Verification items for the finished model (mm, model axes). A direction names the side the tool comes from. Round coordinates to 2 decimals unless told otherwise and drop trailing zeros. Order: outer loops, then holes, each group sorted by start corner. A loop starts at its lowest first (then second) coordinate and runs counter-clockwise, first axis right, second up.
```python
from build123d import *

# Parameters (mm, degrees)
SKETCH1_W           = 104
SKETCH1_H           = 9.72
BODY_DEPTH          = 17.75
FRONT_CUT_OUT_DEPTH = 89.865925518
SKETCH4_R           = 3.5
BOSS_EXTRUDE2_DEPTH = 9.5


with BuildPart() as part:
    # Sketch1 → body (new body)
    with BuildSketch(Plane.XY):
        with Locations((34.530987618, 4.261078665)):
            Rectangle(SKETCH1_W, SKETCH1_H)
    extrude(amount=BODY_DEPTH)

    # Sketch2 → front_cut_out (cut, through all)
    with BuildSketch(Plane.XZ.offset(0.598921335)):
        with BuildLine():
            Line((46.030987618, 17.75), (56.030987618, 14.8))
            Line((56.030987618, 14.8), (80.030987618, 14.8))
            ThreePointArc((80.030987618, 14.8), (85.955987618, 8.875), (80.030987618, 2.95))
            Line((80.030987618, 2.95), (56.030987618, 2.95))
            Line((56.030987618, 2.95), (46.030987618, 0))
            Line((46.030987618, 0), (86.530987618, 0))
            Line((86.530987618, 0), (86.530987618, 17.75))
            Line((86.530987618, 17.75), (46.030987618, 17.75))
        make_face()
    extrude(amount=-FRONT_CUT_OUT_DEPTH, mode=Mode.SUBTRACT)

    # Sketch4 → Boss-Extrude2 (add)
    with BuildSketch(Plane.XZ.offset(0.598921335)):
        with Locations(Location((-8.469012382, 8.875, 0), (0, 0, 180))):
            Circle(SKETCH4_R)
        with Locations(Location((42.530987618, 8.875, 0), (0, 0, 180))):
            Circle(SKETCH4_R)
        with Locations(Location((59.530872729, 9, 0), (0, 0, 180))):
            Circle(SKETCH4_R)
        with Locations(Location((76.530895707, 9, 0), (0, 0, 180))):
            Circle(SKETCH4_R)
    extrude(amount=BOSS_EXTRUDE2_DEPTH)


solid = part.part
```
1) Sectioned sample at D-D on z = 16. Record the cut outline in (x, y), then the cut area to 3 significant figures.
2) Draft check along X on faces 1 (the flat face through (51.101, 4.193, 1.496)), 2 (the cylindrical face through (73.298, -5.282, 10.341)), 3 (the flat face through (43, -10.099, 9)), 4 (the flat face through (-17.469, 4, 9)). Enter one of: released by +X, released by -X, zero draft, split by the parting line, or undercut.
3) Scan lines: probe 1 along X at (y, z) = (-8, 6.75); probe 2 along Y at (x, z) = (53, 12); probe 3 along Z at (x, y) = (42.5, -8.5). Record each from-to range of solid material in increasing order.
4) Sectioned sample at B-B on x = 60.5. Record the cut outline in (y, z), then the cut area to 3 significant figures.
5) Sectioned sample at A-A on y = 6.5. Record the cut outline in (x, z) (3 decimals).
6) Tool access check on faces 5 (the flat face through (68, 4, 14.8)), 6 (the cylindrical face through (39.3, -5.28, 10.22)), 7 (the flat face through (77, -10.099, 9)), 8 (the flat face through (68, 4, 2.95)), 9 (the cylindrical face through (85.955, 4.193, 9.005)). Record the directions out of +Z, -Z, +X, -X, +Y, -Y that give a thin tool (end or side, any length) a straight path to the whole face; none if there is none.
7) Sectioned sample at C-C on y = -1.5. Record the cut outline in (x, z) (3 decimals).
8) Go/stop test with flat-tipped pins: pin 1 Ø5 at (x, y) = (64.5, -0.5) entering from +Z; pin 2 Ø5 at (x, y) = (60, 2) entering from -Z; pin 3 Ø1.5 at (y, z) = (-0.5, 13) entering from +X. Record where each tip stops, or that it passes through.
Returned:
1. outline: (-17.47, -0.6) - (51.96, -0.6) - (51.96, 9.12) - (-17.47, 9.12) - close
1. area: 675 mm2
2. face 1: released by +X
2. face 2: undercut
2. face 3: zero draft
2. face 4: released by -X
3. probe 1: x = -11.25 to -5.69, 39.75 to 45.31, 56.85 to 62.21, 73.85 to 79.21
3. probe 2: y = -0.6 to 9.12
3. probe 3: z = 5.38 to 12.37
4. outline: (-10.1, 5.64) - (-0.6, 5.64) - (-0.6, 2.95) - (9.12, 2.95) - (9.12, 14.8) - (-0.6, 14.8) - (-0.6, 12.36) - (-10.1, 12.36) - close
4. area: 179 mm2
5. outline: (-17.469, 0) - (46.031, 0) - (56.031, 2.95) - (80.031, 2.95) arc R5.925 ccw to (80.031, 14.8) - (56.031, 14.8) - (46.031, 17.75) - (-17.469, 17.75) - close
6. face 5: +Z, +X, +Y, -Y
6. face 6: -Y
6. face 7: +Z, -Z, +X, -X, -Y
6. face 8: -Z, +X, +Y, -Y
6. face 9: +X, +Y, -Y
7. outline: circle Ø7 at (-8.469, 8.875); circle Ø7 at (42.531, 8.875); circle Ø7 at (59.531, 9); circle Ø7 at (76.531, 9)
8. pin 1: stops at z = 14.8
8. pin 2: stops at z = 2.95
8. pin 3: stops at x = 84.9
